```python
from build123d import *

# Parameters (mm, degrees)
F0_R     = 3.302
F0_R_2   = 1.7
F0_R_3   = 18
F1_DEPTH = 12.7
F2_DEPTH = 25.4
F4_R     = 6.35
F3_R     = 1.7
F5_DEPTH = 12.7
F6_R     = 2.7051
F7_DEPTH = 25.4


# Not quite as in the source:
# - a feature names something its author has since deleted; it is built from what else it names


with BuildPart() as f1:
    # F0 (on Front) → F1 (new body)
    with BuildSketch(Plane.XZ):
        with BuildLine():
            Line((108.4265169831, 0.0004552842), (32.2265169831, 152.4004552842))
            Line((32.2265169831, 152.4004552842), (-107.4734830169, 152.4004552842))
            Line((-107.4734830169, 152.4004552842), (-107.4734830169, -76.1995447158))
            add(Edge.make_bspline(
                [(-82.0734830169, -114.2995447158), (-82.8863746009, -95.7832909802), (-85.4194185281, -76.1871889735), (-107.4734830169, -76.1995447158)],
                knots=[0, 0, 0, 0, 45.7905011984, 45.7905011984, 45.7905011984, 45.7905011984], degree=3))
            Line((-82.0734830169, -114.2995447158), (108.4265169831, -114.2995447158))
            Line((108.4265169831, -114.2995447158), (108.4265169831, 0.0004552842))
        make_face()
        with Locations((-88.4234830169, -57.1371889735)):
            Circle(F0_R, mode=Mode.SUBTRACT)
        with Locations((-88.4234830169, -19.0371889735)):
            Circle(F0_R, mode=Mode.SUBTRACT)
        with Locations((-92.9944827628, 14.5430932346)):
            Circle(F0_R_2, mode=Mode.SUBTRACT)
        with Locations((-69.4244827628, 17.1130932346)):
            Circle(F0_R_2, mode=Mode.SUBTRACT)
        with Locations((-45.8544827628, 14.5430932346)):
            Circle(F0_R_2, mode=Mode.SUBTRACT)
        with Locations((-90.4244827628, 38.1130932346)):
            Circle(F0_R_2, mode=Mode.SUBTRACT)
        with Locations((-69.4244827628, 38.1130932346)):
            Circle(F0_R_3, mode=Mode.SUBTRACT)
        with Locations((-92.9944827628, 61.6830932346)):
            Circle(F0_R_2, mode=Mode.SUBTRACT)
        with Locations((-69.4244827628, 59.1130932346)):
            Circle(F0_R_2, mode=Mode.SUBTRACT)
        with Locations((-48.4244827628, 38.1130932346)):
            Circle(F0_R_2, mode=Mode.SUBTRACT)
        with Locations((-45.8544827628, 61.6830932346)):
            Circle(F0_R_2, mode=Mode.SUBTRACT)
        with Locations((-88.4234830169, 95.2504552842)):
            Circle(F0_R, mode=Mode.SUBTRACT)
        with Locations((-88.4234830169, 133.3504552842)):
            Circle(F0_R, mode=Mode.SUBTRACT)
        with Locations((-92.9944827628, 14.5430932346)):
            Circle(F0_R_2)
        with Locations((-45.8544827628, 61.6830932346)):
            Circle(F0_R_2)
    extrude(amount=F1_DEPTH)

    # F0 (on Front) → F2 (cut)
    with BuildSketch(Plane.XZ):
        with BuildLine():
            add(Edge.make_bspline(
                [(-82.0734830169, -114.2995447158), (-82.8863746009, -95.7832909802), (-85.4194185281, -76.1871889735), (-107.4734830169, -76.1995447158)],
                knots=[0, 0, 0, 0, 45.7905011984, 45.7905011984, 45.7905011984, 45.7905011984], degree=3))
            Line((-107.4734830169, -76.1995447158), (-107.4734830169, -114.2995447158))
            Line((-107.4734830169, -114.2995447158), (-82.0734830169, -114.2995447158))
        make_face()
        with BuildLine():
            Line((108.4265169831, 0.0004552842), (32.2265169831, 152.4004552842))
            Line((32.2265169831, 152.4004552842), (-107.4734830169, 152.4004552842))
            Line((-107.4734830169, 152.4004552842), (-107.4734830169, -76.1995447158))
            add(Edge.make_bspline(
                [(-82.0734830169, -114.2995447158), (-82.8863746009, -95.7832909802), (-85.4194185281, -76.1871889735), (-107.4734830169, -76.1995447158)],
                knots=[0, 0, 0, 0, 45.7905011984, 45.7905011984, 45.7905011984, 45.7905011984], degree=3))
            Line((-82.0734830169, -114.2995447158), (108.4265169831, -114.2995447158))
            Line((108.4265169831, -114.2995447158), (108.4265169831, 0.0004552842))
        make_face()
        with Locations((-88.4234830169, -57.1371889735)):
            Circle(F0_R, mode=Mode.SUBTRACT)
        with Locations((-88.4234830169, -19.0371889735)):
            Circle(F0_R, mode=Mode.SUBTRACT)
        with Locations((-92.9944827628, 14.5430932346)):
            Circle(F0_R_2, mode=Mode.SUBTRACT)
        with Locations((-69.4244827628, 17.1130932346)):
            Circle(F0_R_2, mode=Mode.SUBTRACT)
        with Locations((-45.8544827628, 14.5430932346)):
            Circle(F0_R_2, mode=Mode.SUBTRACT)
        with Locations((-90.4244827628, 38.1130932346)):
            Circle(F0_R_2, mode=Mode.SUBTRACT)
        with Locations((-69.4244827628, 38.1130932346)):
            Circle(F0_R_3, mode=Mode.SUBTRACT)
        with Locations((-92.9944827628, 61.6830932346)):
            Circle(F0_R_2, mode=Mode.SUBTRACT)
        with Locations((-69.4244827628, 59.1130932346)):
            Circle(F0_R_2, mode=Mode.SUBTRACT)
        with Locations((-48.4244827628, 38.1130932346)):
            Circle(F0_R_2, mode=Mode.SUBTRACT)
        with Locations((-45.8544827628, 61.6830932346)):
            Circle(F0_R_2, mode=Mode.SUBTRACT)
        with Locations((-88.4234830169, 95.2504552842)):
            Circle(F0_R, mode=Mode.SUBTRACT)
        with Locations((-88.4234830169, 133.3504552842)):
            Circle(F0_R, mode=Mode.SUBTRACT)
    extrude(amount=-F2_DEPTH, mode=Mode.SUBTRACT)

    # F4
    f4_edges = [f1.edges().sort_by_distance(p)[0] for p in [
        (-107.473483, -6.35, -76.199545),
        (-107.473483, -6.35, 152.400455),
        (108.426517, -6.35, 0.000455),
        (32.226517, -6.35, 152.400455),
    ]]
    fillet(f4_edges, radius=F4_R)

    # F3 (on face) → F5 (join)
    with BuildSketch(Plane.XZ.offset(12.7)):
        with Locations((-45.8544827628, 14.5430932346)):
            Circle(F3_R)
        with Locations((-92.9944827628, 61.6830932346)):
            Circle(F3_R)
    extrude(amount=-F5_DEPTH)

    # F6 (on face) → F7 (cut)
    with BuildSketch(Plane(origin=(0, 0, -114.2995447158), x_dir=(1, 0, 0), z_dir=(0, 0, -1))):
        with Locations((-69.3734830169, 6.35)):
            Circle(F6_R)
        with Locations((-28.0984830169, 6.35)):
            Circle(F6_R)
        with Locations((13.1765169831, 6.35)):
            Circle(F6_R)
        with Locations((54.4515169831, 6.35)):
            Circle(F6_R)
        with Locations((95.7265169831, 6.35)):
            Circle(F6_R)
    extrude(amount=-F7_DEPTH, mode=Mode.SUBTRACT)


solid = f1.part
```
The listing builds one solid part. Answer for the finished solid, in the listing's coordinates (mm). A direction names the side the tool comes from. Coordinates: 2 decimals unless noted, no trailing zeros. Write each loop counter-clockwise with the first axis right and the second up, starting at its lowest first coordinate (ties: lowest second). Pieces come first, ordered by that corner, then holes.
Q1. Section C-C, the plane x = 67 is taken. Write down the section's boundary in (y, z).
Returned:
outline: (-12.7, -114.3) - (0, -114.3) - (0, 82.85) - (-12.7, 82.85) - close
Q2. Which of the six approach directions +Z, -Z, +X, -X, +Y, -Y give full straight-line access (tool end or side, diameter ignored) to faces 1 (the cylindrical face through (51.75, -6.47, -101.78)), 2 (the cylindrical face through (-87.407, -6.261, 38.905))?
Returned:
face 1: -Z
face 2: +Y, -Y
Q3. Section B-B, the plane y = -6.35 is taken. Give the number of separate pieces and of enclosed holes in the cut face, then the cut area to 3 significant figures.
Returned:
separate pieces: 1
enclosed holes: 9
area: 49,100 mm2
Q4. Find the intervals of material crossed by line 1 along X through (y, z) = (-6.35, -95.25); line 2 along X through (y, z) = (-8.75, -94); line 3 along Z through (x, y) = (-77, -2.5), in increasing order.
Returned:
line 1: x = -84.35 to -72.08, -66.67 to -30.8, -25.39 to 10.47, 15.88 to 51.75, 57.16 to 93.02, 98.43 to 108.43
line 2: x = -84.68 to -70.62, -68.13 to -29.35, -26.85 to 11.93, 14.42 to 53.2, 55.7 to 94.48, 96.97 to 108.43
line 3: z = -114.3 to 21.78, 54.44 to 152.4
Q5. The mould has two halves that part along Y. Classify faces 3 (the flat face through (-1, 0, 21)), 4 (the flat face through (13, -6, -88.9)), 5 (the cylindrical face through (-105.564, -6.439, 150.59)): released by +Y, released by -Y, zero draft, split by the parting line, or undercut.
Returned:
face 3: released by +Y
face 4: undercut
face 5: zero draft
Q6. Section D-D, the plane z = 82 is taken. Write down the section's boundary in (x, y), then the cut area to 3 significant figures.
Returned:
outline: (-107.47, -12.7) - (67.43, -12.7) - (67.43, 0) - (-107.47, 0) - close
area: 2,220 mm2
Q7. Given P1, Ø1.6, axis at x = 55.5, y = -6, coming from the -Z side, flat-ended and moving along its own axis, determine where the tip first touches the part or whether it passes through.
Returned:
P1: stops at z = -88.9
Q8. Section A-A, the plane z = 49 is taken. Write down the section's boundary in (x, y).
Returned:
outline: (-107.47, -12.7) - (-83.76, -12.7) - (-83.76, 0) - (-107.47, 0) - close; (-55.09, -12.7) - (83.93, -12.7) - (83.93, 0) - (-55.09, 0) - close
